```python
from build123d import *

# Parameters (mm, degrees)
F1_DEPTH    = 116.84
F2_W        = 86.36
F2_H        = 15.24
F3_DEPTH    = 2.54
F4_W        = 86.36
F4_H        = 15.24
F5_DEPTH    = 2.54
F6_T1_DEPTH = 148.0482991577
F6_T3_DEPTH = 112.4882991577
F7_SIZE     = 5.08
F8_W        = 91.7793288827
F8_H        = 30.2478149533
F9_DEPTH    = 106.68
F10_W       = 99.2863364518
F10_H       = 25.3497036174
F11_DEPTH   = 10.16
F12_W       = 15.3326203581
F12_H       = 21.305212751
F13_DEPTH   = 43.18


# Not quite as in the source:
# - a fillet or chamfer that OpenCascade refuses, or shapes differently, is made with other operations: its cross-section is extruded or revolved along the edge and cut away or added


with BuildPart() as f1:
    # F0 (on Front) → F1 (new body)
    with BuildSketch(Plane.XZ):
        Polygon((43.18, 0), (36.83, 0), (29.21, -13.1982271537), (13.97, -13.1982271537), (6.35, 0), (0, 0), (-6.35, 0), (-13.97, -13.1982271537), (-29.21, -13.1982271537), (-36.83, 0), (-43.18, 0), (-43.18, -15.24), (0, -15.24), (43.18, -15.24), align=None)
    extrude(amount=F1_DEPTH)

    # F2 (on face) → F3 (join)
    with BuildSketch(Plane.XZ.offset(116.84)):
        with Locations((0, -7.62)):
            Rectangle(F2_W, F2_H)
    extrude(amount=F3_DEPTH)

    # F4 (on face) → F5 (join)
    with BuildSketch(Plane(origin=(0, 0, 0), x_dir=(-1, 0, 0), z_dir=(0, 1, 0))):
        with Locations((0, -7.62)):
            Rectangle(F4_W, F4_H)
    extrude(amount=F5_DEPTH)

    # F6: chamfer of 5.08 on 4 edges, made by hand

    # F6_s2 → F6_t1 (cut)
    with BuildSketch(Plane.XZ.offset(-15.6041495789)):
        Polygon((-38.1, 0), (-43.18, -5.08), (-43.18, 0), align=None)
        Polygon((38.1, 0), (43.18, -5.08), (43.18, 0), align=None)
    extrude(amount=F6_T1_DEPTH, mode=Mode.SUBTRACT)

    # F6_s4 → F6_t3 (cut)
    with BuildSketch(Plane.YZ.offset(-56.2441495789)):
        Polygon((-114.3, 0), (-119.38, -5.08), (-119.38, 0), align=None)
        Polygon((-2.54, 0), (2.54, -5.08), (2.54, 0), align=None)
    extrude(amount=F6_T3_DEPTH, mode=Mode.SUBTRACT)

    # F7
    f7_edges = [f1.edges().sort_by_distance(p)[0] for p in [
        (-43.18, -119.38, -10.16),
        (43.18, -119.38, -10.16),
        (43.18, 2.54, -10.16),
        (-43.18, 2.54, -10.16),
    ]]
    chamfer(f7_edges, length=F7_SIZE)

    # F8 (on face) → F9 (cut)
    with BuildSketch(Plane.XZ.offset(119.38)):
        with Locations((-0.610165298, -4.9024894834)):
            Rectangle(F8_W, F8_H)
    extrude(amount=-F9_DEPTH, mode=Mode.SUBTRACT)

    # F10 (on face) → F11 (cut)
    with BuildSketch(Plane(origin=(0, 2.54, 0), x_dir=(-1, 0, 0), z_dir=(0, 1, 0))):
        with Locations((1.3202968985, -7.6577230357)):
            Rectangle(F10_W, F10_H)
    extrude(amount=-F11_DEPTH, mode=Mode.SUBTRACT)

    # F12 (on face) → F13 (cut)
    with BuildSketch(Plane(origin=(-43.18, 0, 0), x_dir=(0, -1, 0), z_dir=(-1, 0, 0))):
        with Locations((10.5058533372, -7.6547963545)):
            Rectangle(F12_W, F12_H)
    extrude(amount=-F13_DEPTH, mode=Mode.SUBTRACT)


solid = f1.part
```
Can you work these out from the model? Positions are in its coordinate system, mm. A direction names the side the tool comes from. Coordinates: 2 decimals unless noted, no trailing zeros. Loops run counter-clockwise (first coordinate to the right, second up) from the corner with the lowest first, then second, coordinate; pieces in that order, holes last. Notation, with made-up numbers: (75, -26) -> (89, -26) arc R14 ccw to (89, 1) -> close; hole circle Ø1 at (71, 45.25). An arc over 180 degrees is marked (long way). Answer as a JSON object with one key per item and string values.
1) Imagine slicing it at D-D (z = -10.25). Please give me the cut outline in (x, y).
Results:
{"outline": "(0, -12.7) -> (12.27, -12.7) -> (12.27, -7.62) -> (0, -7.62) -> close; (30.91, -12.7) -> (43.18, -12.7) -> (43.18, -7.62) -> (30.91, -7.62) -> close"}
2) Imagine slicing it at C-C (x = 28.5). Please give me the cut outline in (y, z).
Results:
{"outline": "(-12.7, -15.24) -> (-7.62, -15.24) -> (-7.62, -13.2) -> (-12.7, -13.2) -> close"}
3) For P1, Ø3, axis at x = 24, y = -11.5, coming from the +Z side, with a flat end and sliding along its axis, tell me the tip position at first contact or that it passes through.
Results:
{"P1": "stops at z = -13.2"}
4) Thinking about a two-plate mould opening in X: for faces 1 (the face through (22, -10, -15.24)), 2 (the face through (43.18, -10, -10)), 3 (the face through (22, -10, -13.198)), which applies, pulls with the +X half, pulls with the -X half, needs draft (parallel to the pull), parting line crosses it, or undercut?
Results:
{"face 1": "needs draft", "face 2": "pulls with the +X half", "face 3": "undercut"}
5) Imagine slicing it at A-A (z = -3.5). Please give me the cut outline in (x, y).
Results:
{"outline": "(0, -12.7) -> (8.37, -12.7) -> (8.37, -7.62) -> (0, -7.62) -> close; (34.81, -12.7) -> (41.6, -12.7) -> (41.6, -7.62) -> (34.81, -7.62) -> close"}
6) Imagine slicing it at B-B (y = -11.7). Please give me the cut outline in (x, z).
Results:
{"outline": "(0, -15.24) -> (43.18, -15.24) -> (43.18, -5.08) -> (38.1, 0) -> (36.83, 0) -> (29.21, -13.2) -> (13.97, -13.2) -> (6.35, 0) -> (0, 0) -> close"}
7) For faces 4 (the face through (21, -12.7, -14)), 5 (the face through (10.213, -10.124, -6.692)), which set-ups out of +Z, -Z, +X, -X, +Y, -Y let a thin tool reach every point of the face, with its end or its side?
Results:
{"face 4": "+Z, -Z, +X, -X, -Y", "face 5": "+Z, +Y, -Y"}
8) If I drill on line 1 (Z direction, x = 19, y = -8.25); line 2 (X direction, y = -8.6, z = -5.75); line 3 (X direction, y = -9.15, z = -8.75), over which ranges is the centre line in solid material (lowest first)?
Results:
{"line 1": "z = -15.24 to -13.2", "line 2": "x = 0 to 9.67, 33.51 to 43.18", "line 3": "x = 0 to 11.4, 31.78 to 43.18"}
